from build123d import *

# Parameters (mm, degrees)
SKETCH1_W           = 122
SKETCH1_H           = 25
SKETCH1_R           = 1.5
BOSS_EXTRUDE1_DEPTH = 12.5
BOSS_EXTRUDE2_DEPTH = 25


with BuildPart() as part:
    # Sketch1 → Boss-Extrude1 (new body)
    with BuildSketch(Plane(origin=(0, 0, 0), x_dir=(0, 0, -1), z_dir=(1, 0, 0))):
        with Locations((61, 12.5)):
            Rectangle(SKETCH1_W, SKETCH1_H)
        with Locations((5, 20)):
            Circle(SKETCH1_R, mode=Mode.SUBTRACT)
        with Locations((17, 20)):
            Circle(SKETCH1_R, mode=Mode.SUBTRACT)
        with Locations((17, 5)):
            Circle(SKETCH1_R, mode=Mode.SUBTRACT)
        with Locations((5, 5)):
            Circle(SKETCH1_R, mode=Mode.SUBTRACT)
    extrude(amount=-BOSS_EXTRUDE1_DEPTH)

    # Sketch2 → Boss-Extrude2 (add)
    with BuildSketch(Plane(origin=(0, 25, 0), x_dir=(1, 0, 0), z_dir=(0, 1, 0))):
        Polygon((-12.5, 122), (-25, 22), (-12.5, 22), align=None)
    extrude(amount=-BOSS_EXTRUDE2_DEPTH)


solid = part.part
Build history of the part. All positions in model axes, mm. A direction names the side the tool comes from. Round coordinates to 2 decimals unless told otherwise and drop trailing zeros. Write each loop counter-clockwise with the first axis right and the second up, starting at its lowest first coordinate (ties: lowest second). Pieces come first, ordered by that corner, then holes. Notation, with made-up numbers: (54.25, 40.25) - (58.25, 40.25) arc R36 cw to (58.25, 76.25) - close; hole circle Ø3 at (-33.75, -36). An arc over 180 degrees is marked (long way). One line per question, with ' | ' between items.
1. Band-saw the part on A-A, the plane z = -17. Write the cut outline in (x, y).
Results are:
outline: (-12.5, 0) - (0, 0) - (0, 3.5) - (-12.5, 3.5) - close; (-12.5, 6.5) - (0, 6.5) - (0, 18.5) - (-12.5, 18.5) - close; (-12.5, 21.5) - (0, 21.5) - (0, 25) - (-12.5, 25) - close
2. Band-saw the part on C-C, the plane x = -21. Write the cut outline in (y, z).
Results are:
outline: (0, -54) - (25, -54) - (25, -22) - (0, -22) - close
3. Band-saw the part on B-B, the plane y = 5. Write the cut outline in (x, z).
Results are:
outline: (-25, -22) - (-12.5, -122) - (0, -122) - (0, -18.5) - (-12.5, -18.5) - (-12.5, -22) - close; (-12.5, -15.5) - (0, -15.5) - (0, -6.5) - (-12.5, -6.5) - close; (-12.5, -3.5) - (0, -3.5) - (0, 0) - (-12.5, 0) - close
4. Band-saw the part on D-D, the plane y = 23. Write the cut outline in (x, z).
Results are:
outline: (-25, -22) - (-12.5, -122) - (0, -122) - (0, 0) - (-12.5, 0) - (-12.5, -22) - close
5. Tool access for faces 5 (the face through (-6.16, 21.01, -15.89)), 6 (the face through (-19, 13, -22)): list every direction of +Z, -Z, +X, -X, +Y, -Y with a clear straight run to the whole face (end or side of a thin tool).
Results are:
face 5: +X, -X | face 6: +Z, -X, +Y, -Y
6. Drop flat-ended pins along their axis: pin 1 Ø12 at (x, y) = (-15, 7) entering from -Z; pin 2 Ø3.5 at (y, z) = (5, -17) entering from -X; pin 3 Ø1.8 at (y, z) = (5, -5) entering from +X; pin 4 Ø12 at (y, z) = (22, -67) entering from -X (3 decimals). Give the stop position or say it passes through.
Results are:
pin 1: z = -122 | pin 2: x = -12.5 | pin 3: through | pin 4: x = -20.125
7. Drill centre lines: line 1 along Y through (x, z) = (-3.25, -17); line 2 along Z through (x, y) = (-12, 19); line 3 along X through (y, z) = (14.75, -11.5). Where is each one in solid material? Low to high. Write a range as from..to.
Results are:
line 1: 0..3.5, 6.5..18.5, 21.5..25 | line 2: -122..-18.12, -15.88..-6.12, -3.88..0 | line 3: -12.5..0
8. Mould opens along Z. For faces 1 (the face through (-6.162, 4.425, -6.386)), 2 (the face through (-10, 25, -62)), 3 (the face through (-18.662, 12.675, -72.7)), 4 (the face through (-6, 12, 0)) say: released by +Z, released by -Z, zero draft, split by the parting line, or undercut.
Results are:
face 1: undercut | face 2: zero draft | face 3: released by -Z | face 4: released by +Z
